Read the model definition and answer for the solid it produces. Units are mm, in the model's axes. Round coordinates to 2 decimals unless told otherwise and drop trailing zeros. Write each loop counter-clockwise with the first axis right and the second up, starting at its lowest first coordinate (ties: lowest second). Pieces come first, ordered by that corner, then holes. Notation, with made-up numbers: (-1, -38) - (9, -38) arc R15 ccw to (9, -16) - close; hole circle Ø8 at (17, -4). An arc over 180 degrees is marked (long way). Answer as CSV lines item,"result". Start each with the question number.
1) Each of these flat-tipped pins is pushed along its axis until it touches: pin 1 (1.2 mm diameter, centred on x = -41.14, z = -23.75, fed in from +Y) (3 decimals); pin 2 (1 mm diameter, centred on x = -23, y = 2, fed in from -Z). Where does it stop, or does it pass through?
2) Find section B-B on z = 29.5. Determine the outline of the cut face in (x, y), then the cut area to 3 significant figures.
3) For a pull along Z with two mould halves and no side action, classify faces 1 (the flat face through (1, 2, 10)), 2 (the cylindrical face through (33.454, 0.986, -36.484)), 3 (the cylindrical face through (-7.81, 0.99, -1.73)) as +Z half, -Z half, draft (parallel to the pull), parting line (faces both ways), or undercut.
4) Consider line 1 along X through (y, z) = (1.2, 23.75); line 2 along X through (y, z) = (0.65, 0); line 3 along Z through (x, y) = (26, 0.9). Determine where each line is inside the solid, lowest interval first.
5) Find section C-C on x = -18. Determine the outline of the cut face in (y, z), then the cut area to 3 significant figures.
6) Find section A-A on y = 1.5. State how many separate pieces and enclosed holes the cut face has, then the cut area to 3 significant figures.
from build123d import *

# Parameters (mm, degrees)
SKETCH1_R               = 49.5
SKETCH1_R_2             = 8
SKETCH1_R_3             = 1
BOSS_EXTRUDE1_DEPTH     = 2
CUT_EXTRUDE1_DEPTH      = 71.032135481
CUT_EXTRUDE1_DEPTH_BACK = 71.032135481
SKETCH2_R               = 0.42
SKETCH3_R               = 1
CUT_EXTRUDE2_DEPTH      = 1


with BuildPart() as part:
    # Sketch1 → Boss-Extrude1 (new body)
    with BuildSketch(Plane(origin=(0, 0, 0), x_dir=(1, 0, 0), z_dir=(0, 1, 0))):
        with Locations(Location((0, 0, 0), (0, 0, 270))):
            Circle(SKETCH1_R)
        with Locations(Location((0, 0, 0), (0, 0, 270))):
            Circle(SKETCH1_R_2, mode=Mode.SUBTRACT)
        with Locations(Location((0, 47.5, 0), (0, 0, 270))):
            Circle(SKETCH1_R_3, mode=Mode.SUBTRACT)
        with Locations(Location((41.13620668, 23.75, 0), (0, 0, 270))):
            Circle(SKETCH1_R_3, mode=Mode.SUBTRACT)
        with Locations(Location((41.13620668, -23.75, 0), (0, 0, 270))):
            Circle(SKETCH1_R_3, mode=Mode.SUBTRACT)
        with Locations(Location((0, -47.5, 0), (0, 0, 270))):
            Circle(SKETCH1_R_3, mode=Mode.SUBTRACT)
        with Locations(Location((-41.13620668, -23.75, 0), (0, 0, 270))):
            Circle(SKETCH1_R_3, mode=Mode.SUBTRACT)
        with Locations(Location((-41.13620668, 23.75, 0), (0, 0, 270))):
            Circle(SKETCH1_R_3, mode=Mode.SUBTRACT)
    extrude(amount=BOSS_EXTRUDE1_DEPTH)

    # Sketch2 → Cut-Extrude1 (cut, two sides: drawn at the far end of the back side and taken through both)
    with BuildSketch(Plane(origin=(0, 2, 0), x_dir=(1, 0, 0), z_dir=(0, 1, 0)).offset(-CUT_EXTRUDE1_DEPTH_BACK)):
        with Locations(Location((0, 21, 0), (0, 0, 270))):
            Circle(SKETCH2_R)
    extrude(amount=CUT_EXTRUDE1_DEPTH + CUT_EXTRUDE1_DEPTH_BACK, mode=Mode.SUBTRACT)

    # Sketch3 → Cut-Extrude2 (cut)
    with BuildSketch(Plane.XZ):
        with Locations(Location((-6.15636258, 16.914467174, 0), (0, 0, 270))):
            Circle(SKETCH3_R)
        with Locations(Location((-6.15636258, -16.914467174, 0), (0, 0, 270))):
            Circle(SKETCH3_R)
        with Locations(Location((18, 0, 0), (0, 0, 270))):
            Circle(SKETCH3_R)
    extrude(amount=-CUT_EXTRUDE2_DEPTH, mode=Mode.SUBTRACT)


solid = part.part
Check values:
1,pin 1,"passes through"
1,pin 2,"stops at z = -44.09"
2,outline,"(-39.75, 0) - (39.75, 0) - (39.75, 2) - (-39.75, 2) - close"
2,area,"159 mm^2"
3,face 1,"draft"
3,face 2,"parting line"
3,face 3,"undercut"
4,line 1,"x = -43.43 to -42.14, -40.14 to 40.14, 42.14 to 43.43"
4,line 2,"x = -49.5 to -8, 8 to 17, 19 to 49.5"
4,line 3,"z = -42.12 to 42.12"
5,outline,"(0, -46.11) - (2, -46.11) - (2, 46.11) - (0, 46.11) - close"
5,area,"184 mm^2"
6,separate pieces,"1"
6,enclosed holes,"8"
6,area,"7,480 mm^2"
